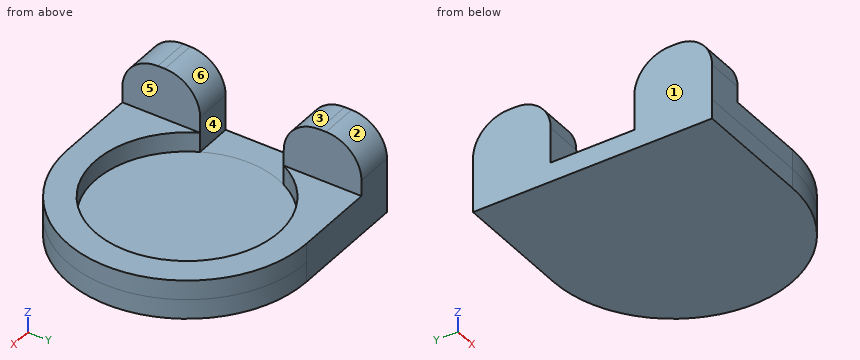
from build123d import *

# Parameters (mm, degrees)
F0_R      = 32.9
F1_DEPTH  = 25.4
F1_FACE_R = 32.9
F2_R      = 32.9
F3_DEPTH  = 7
F5_DEPTH  = 25.4
F7_DEPTH  = 18.4
F8_R      = 12.7


with BuildPart() as f1:
    # F0 (on Top) → F1 (new body)
    with BuildSketch(Plane.XY):
        with BuildLine():
            ThreePointArc((-42.9, 1.789e-07), (-30.3348808497, 30.3348809761), (0, 42.9))
            Line((0, 42.9), (-42.9, 42.9))
            Line((-42.9, 42.9), (-42.9, 1.789e-07))
        make_face()
        with BuildLine():
            Line((-42.9, -42.9), (0, -42.9))
            ThreePointArc((0, -42.9), (-30.3348809761, -30.3348808497), (-42.9, 1.789e-07))
            Line((-42.9, 1.789e-07), (-42.9, -42.9))
        make_face()
        with BuildLine():
            ThreePointArc((0, -42.9), (30.3348809129, -30.3348809129), (42.9, 0))
            ThreePointArc((42.9, 0), (30.3348809129, 30.3348809129), (0, 42.9))
            ThreePointArc((0, 42.9), (-30.3348808497, 30.3348809761), (-42.9, 1.789e-07))
            ThreePointArc((-42.9, 1.789e-07), (-30.3348809761, -30.3348808497), (0, -42.9))
        make_face()
        Circle(F0_R, mode=Mode.SUBTRACT)
    extrude(amount=F1_DEPTH)

    # F1_face (on face) + F2 (on Top) → F3 (join)
    with BuildSketch(Plane(origin=(-8.2989240486, 0, 0), x_dir=(1, 0, 0), z_dir=(0, 0, -1))):
        with BuildLine():
            Line((-34.6010759514, -42.9), (8.2989240486, -42.9))
            ThreePointArc((8.2989240486, -42.9), (51.1989240486, 0), (8.2989240486, 42.9))
            Line((8.2989240486, 42.9), (-34.6010759514, 42.9))
            Line((-34.6010759514, 42.9), (-34.6010759514, -42.9))
        make_face()
        with Locations((8.2989240486, 0)):
            Circle(F1_FACE_R, mode=Mode.SUBTRACT)
    with BuildSketch(Plane.XY):
        Circle(F2_R)
    extrude(amount=F3_DEPTH, dir=(0, 0, -1))

    # F4 (on Top) → F5 (cut)
    with BuildSketch(Plane.XY):
        with BuildLine():
            ThreePointArc((-29.2815641659, -15), (-32.9, 0), (-29.2815641659, 15))
            Line((-29.2815641659, 15), (-42.9, 15))
            Line((-42.9, 15), (-42.9, -15))
            Line((-42.9, -15), (-29.2815641659, -15))
        make_face()
    extrude(amount=F5_DEPTH, mode=Mode.SUBTRACT)

    # F6 (on face) → F7 (cut)
    with BuildSketch(Plane.XY.offset(25.4)):
        with BuildLine():
            Line((-29.2815641659, 42.9), (-29.2815641659, 15))
            ThreePointArc((-29.2815641659, 15), (32.9, 0), (-29.2815641659, -15))
            Line((-29.2815641659, -15), (-29.2815641659, -42.9))
            Line((-29.2815641659, -42.9), (0, -42.9))
            ThreePointArc((0, -42.9), (42.9, 0), (0, 42.9))
            Line((0, 42.9), (-29.2815641659, 42.9))
        make_face()
    extrude(amount=-F7_DEPTH, mode=Mode.SUBTRACT)

    # F8
    f8_edges = [f1.edges().sort_by_distance(p)[0] for p in [
        (-36.090782, -42.9, 25.4),
        (-36.090782, -15, 25.4),
        (-36.090782, 15, 25.4),
        (-36.090782, 42.9, 25.4),
    ]]
    fillet(f8_edges, radius=F8_R)


solid = f1.part
The model under review builds one solid part; all positions refer to its coordinate system, in mm. Face numbers are marked on the shaded views. A direction names the side the tool comes from. Give positions to 0.01 mm unless a question says otherwise; leave off trailing zeros. Order: outer loops, then holes, each group sorted by start corner. A loop starts at its lowest first (then second) coordinate and runs counter-clockwise, first axis right, second up. Notation, with made-up numbers: M 4,35.25 L 37,35.25 A19 ccw 37,41.25 Z; hole C -21,77.5 d1. An arc over 180 degrees is marked long. One line per question, with ' | ' between items. Start each with the question number.
1) Consider section C-C, the plane y = 5.5. Give the boundary of the cut face in (x, z).
2) Consider section A-A, the plane x = 10.5. Give the boundary of the cut face in (y, z).
3) Mouldability with a two-part tool opening along Y and no side actions: class the marked faces 1, 2 and 3 as pulls with the +Y half, pulls with the -Y half, needs draft (parallel to the pull), parting line crosses it, or undercut.
4) Consider section D-D, the plane z = -3. Give the boundary of the cut face in (x, y), then the cut area to 3 significant figures.
5) Consider section B-B, the plane z = 15.5. Give the boundary of the cut face in (x, y), then the cut area to 3 significant figures.
6) For the marked faces 4, 5 and 6, list the 3-axis set-ups (+Z, -Z, +X, -X, +Y, -Y) from which the entire face can be reached by the end or side of a thin tool; tool diameter is ignored.
7) Wall thickness on L1, parallel to Z at x = -34, y = 13; L2, parallel to X at y = -23.5, z = 24; L3, parallel to Y at x = -17, z = 5.5: over which ranges is each line inside the solid? List them lowest first. Write a range as from..to.
8) Clearance check with flat-ended pins moving along their axes: P1, Ø7, axis at x = -35.5, y = -2.5, coming from the +Z side; P2, Ø14.5, axis at y = -23.5, z = 15, coming from the +X side. State where each tip first meets the part, or that it passes through.
Found:
1) outline: M -42.9,-7 L 42.55,-7 L 42.55,7 L 32.44,7 L 32.44,0 L -42.9,0 Z
2) outline: M -41.6,-7 L 41.6,-7 L 41.6,7 L 31.18,7 L 31.18,0 L -31.18,0 L -31.18,7 L -41.6,7 Z
3) face 1: needs draft | face 2: pulls with the +Y half | face 3: undercut
4) outline: M -42.9,-42.9 L 0,-42.9 A42.9 ccw 0,42.9 L -42.9,42.9 Z | area: 6,570 mm²
5) outline: M -42.9,-42.59 L -29.28,-42.59 L -29.28,-15.31 L -42.9,-15.31 Z; M -42.9,15.31 L -29.28,15.31 L -29.28,42.59 L -42.9,42.59 Z | area: 743 mm²
6) face 4: +Z, -X | face 5: +Z, +X, +Y, -Y | face 6: +Z, +X, -X
7) L1: z = -7..0 | L2: x = -42.9..-29.28 | L3: y = -42.9..-28.17, 28.17..42.9
8) P1: stops at z = 0 | P2: stops at x = -29.28
